Geometry: see drawing. Coordinates: mm, zero at the bounding-box minimum. A direction names the side the tool comes from. Round coordinates to 2 decimals unless told otherwise and drop trailing zeros. Loops run counter-clockwise (first coordinate to the right, second up) from the corner with the lowest first, then second, coordinate; pieces in that order, holes last. Notation, with made-up numbers: M 51,34.25 L 71,34.25 A15 ccw 71,39.25 Z; hole C 26.25,-24.75 d3. An arc over 180 degrees is marked long. Answer as a JSON object with one key per item and string values.
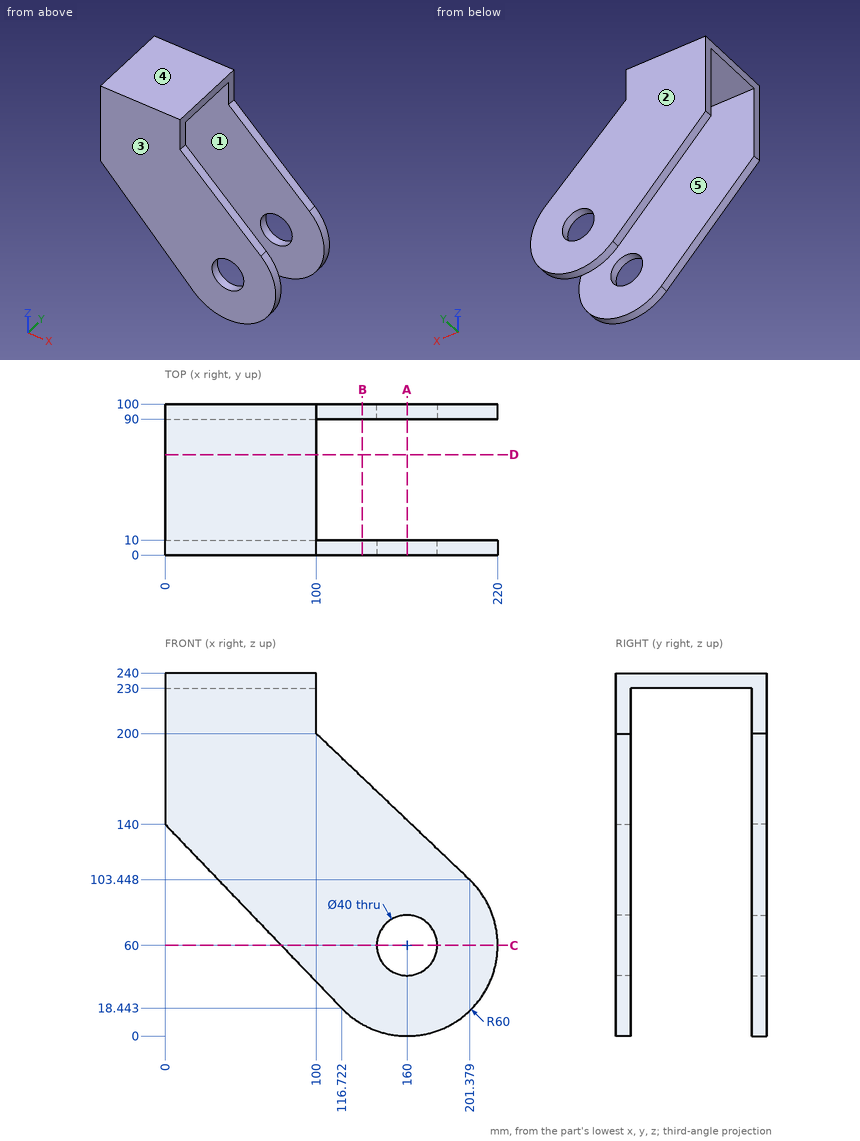
1) Pin query (flat end, axial travel): P1, Ø1.5, axis at x = 93.5, y = 14.5, coming from the -Z side; P2, Ø4, axis at x = 176, z = 49.5, coming from the +Y side; P3, Ø5, axis at x = 186.5, z = 123.5, coming from the +Y side. Return the tip coordinate at first contact, or that it passes through.
Results:
{"P1": "z = 230", "P2": "y = 100", "P3": "through"}
2) Section query B-B (x = 130.5). Return the cut outline in (y, z).
Results:
{"outline": "M 0,7.75 L 10,7.75 L 10,170.95 L 0,170.95 Z; M 90,7.75 L 100,7.75 L 100,170.95 L 90,170.95 Z"}
3) Section query C-C (z = 60). Return the cut outline in (x, y), and give its area (3 significant figures).
Results:
{"outline": "M 76.82,0 L 140,0 L 140,10 L 76.82,10 Z; M 76.82,90 L 140,90 L 140,100 L 76.82,100 Z; M 180,0 L 220,0 L 220,10 L 180,10 Z; M 180,90 L 220,90 L 220,100 L 180,100 Z", "area": "2,060 mm2"}
4) Pull-direction query (Y, two-part tool) for the marked faces 3, 4 and 5; classes: +Y half, -Y half, draft (parallel to the pull), parting line (faces both ways), or undercut.
Results:
{"face 3": "-Y half", "face 4": "draft", "face 5": "undercut"}
5) Section query A-A (x = 160). Return the cut outline in (y, z).
Results:
{"outline": "M 0,0 L 10,0 L 10,40 L 0,40 Z; M 0,80 L 10,80 L 10,142.86 L 0,142.86 Z; M 90,0 L 100,0 L 100,40 L 90,40 Z; M 90,80 L 100,80 L 100,142.86 L 90,142.86 Z"}
6) Ray query, line 1 (Y direction, x = 135.5, z = 97); line 2 (Z direction, x = 38, y = 27); line 3 (X direction, y = 96, z = 60). Return the intervals inside material, ascending.
Results:
{"line 1": "0 to 10, 90 to 100", "line 2": "230 to 240", "line 3": "76.82 to 140, 180 to 220"}
7) Reachability of the marked faces 1 and 2 from +Z, -Z, +X, -X, +Y, -Y: full face, straight path, thin tool, end or side. Return the list, or none.
Results:
{"face 1": "-Z, +X, -X", "face 2": "+Z, -Z, +X, -X, +Y"}
8) Section query D-D (y = 66.5). Return the cut outline in (x, z).
Results:
{"outline": "M 0,230 L 100,230 L 100,240 L 0,240 Z"}
